Read the model definition and answer for the solid it produces. Units are mm, in the model's axes. Coordinates: 2 decimals unless noted, no trailing zeros.
Q1. Section A-A (x = 202) is taken. Count the separate pieces of the cut face and the enclosed holes in it, then the cut area to 3 significant figures.
Q2. Straight lines are drawn through the part: line 1 (Z direction, x = 544, y = 18); line 2 (Z direction, x = 88.5, y = -17); line 3 (Z direction, x = 320, y = 0). For each, find the intervals that lie inside material, in ascending order.
Q3. Flat-ended cylindrical pins translate along their axes: P1, Ø1, axis at x = 490.5, z = -3.5, coming from the +Y side; P2, Ø1.2, axis at x = 401.5, z = 1, coming from the +Y side. Find the tip coordinate at first contact, or state that the pin passes through.
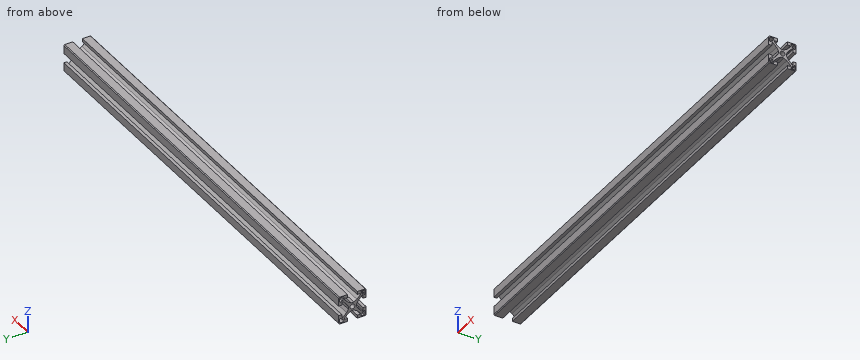
Autodesk Inventor part; units mm, degrees
ref_plane "CS_ANBAU_HINTEN_LINKS_XY" through (670, 0, 20) normal (1, 0, 0) x (0, 0, -1)
ref_plane "CS_ANBAU_HINTEN_LINKS_YZ" through (670, 0, 20) normal (0, 0, -1) x (0, 1, 0)
ref_plane "CS_ANBAU_HINTEN_LINKS_ZX" through (670, 0, 20) normal (0, 1, 0) x (1, 0, 0)
sketch "Skizze_1" plane through (0, 0, 0) normal (1, 0, 0) x (0, 1, 0)
  line L0 (18.75, 20) -> (7, 20)
  line L1 (7, 20) -> (7, 15.5)
  line L2 (7, 15.5) -> (11.7, 15.5)
  line L3 (11.7, 15.5) -> (11.7, 13.82)
  line L4 (11.7, 13.82) -> (6.4481, 8.5681)
  line L5 (6.4481, 8.5681) -> (2, 6)
  line L6 (2, 6) -> (-2, 6)
  line L7 (-2, 6) -> (-6.4481, 8.5681)
  line L8 (-6.4481, 8.5681) -> (-11.7, 13.82)
  line L9 (-11.7, 13.82) -> (-11.7, 15.5)
  line L10 (-11.7, 15.5) -> (-7, 15.5)
  line L11 (-7, 15.5) -> (-7, 20)
  line L12 (-7, 20) -> (-18.75, 20)
  line L13 (-18.75, 20) -> (-20, 18.75)
  line L14 (-20, 18.75) -> (-20, 7)
  line L15 (-20, 7) -> (-15.5, 7)
  line L16 (-15.5, 7) -> (-15.5, 11.7)
  line L17 (-15.5, 11.7) -> (-13.82, 11.7)
  line L18 (-13.82, 11.7) -> (-8.5681, 6.4481)
  line L19 (-8.5681, 6.4481) -> (-6, 2)
  line L20 (-6, 2) -> (-6, -2)
  line L21 (-6, -2) -> (-8.5681, -6.4481)
  line L22 (-8.5681, -6.4481) -> (-13.82, -11.7)
  line L23 (-13.82, -11.7) -> (-15.5, -11.7)
  line L24 (-15.5, -11.7) -> (-15.5, -7)
  line L25 (-15.5, -7) -> (-20, -7)
  line L26 (-20, -7) -> (-20, -18.75)
  line L27 (-20, -18.75) -> (-18.75, -20)
  line L28 (-18.75, -20) -> (-7, -20)
  line L29 (-7, -20) -> (-7, -15.5)
  line L30 (-7, -15.5) -> (-11.7, -15.5)
  line L31 (-11.7, -15.5) -> (-11.7, -13.82)
  line L32 (-11.7, -13.82) -> (-6.4481, -8.5681)
  line L33 (-6.4481, -8.5681) -> (-2, -6)
  line L34 (-2, -6) -> (2, -6)
  line L35 (2, -6) -> (6.4481, -8.5681)
  line L36 (6.4481, -8.5681) -> (11.7, -13.82)
  line L37 (11.7, -13.82) -> (11.7, -15.5)
  line L38 (11.7, -15.5) -> (7, -15.5)
  line L39 (7, -15.5) -> (7, -20)
  line L40 (7, -20) -> (18.75, -20)
  line L41 (18.75, -20) -> (20, -18.75)
  line L42 (20, -18.75) -> (20, -7)
  line L43 (20, -7) -> (15.5, -7)
  line L44 (15.5, -7) -> (15.5, -11.7)
  line L45 (15.5, -11.7) -> (13.82, -11.7)
  line L46 (13.82, -11.7) -> (8.5681, -6.4481)
  line L47 (8.5681, -6.4481) -> (6, -2)
  line L48 (6, -2) -> (6, 2)
  line L49 (6, 2) -> (8.5681, 6.4481)
  line L50 (8.5681, 6.4481) -> (13.82, 11.7)
  line L51 (13.82, 11.7) -> (15.5, 11.7)
  line L52 (15.5, 11.7) -> (15.5, 7)
  line L53 (15.5, 7) -> (20, 7)
  line L54 (20, 7) -> (20, 18.75)
  line L55 (20, 18.75) -> (18.75, 20)
  line L56 (17.75, -12.1) -> (17.1, -12.1)
  line L57 (17.1, -12.1) -> (15.45, -13.75)
  line L58 (15.45, -13.75) -> (14.5, -13.75)
  arc A0 (14.5, -13.75) -> (13.75, -14.5) centre (14.5, -14.5) ccw
  line L59 (13.75, -14.5) -> (13.75, -15.45)
  line L60 (13.75, -15.45) -> (12.1, -17.1)
  line L61 (12.1, -17.1) -> (12.1, -17.75)
  arc A1 (12.1, -17.75) -> (12.85, -18.5) centre (12.85, -17.75) ccw
  line L62 (12.85, -18.5) -> (17.5, -18.5)
  arc A2 (17.5, -18.5) -> (18.5, -17.5) centre (17.5, -17.5) ccw
  line L63 (18.5, -17.5) -> (18.5, -12.85)
  arc A3 (18.5, -12.85) -> (17.75, -12.1) centre (17.75, -12.85) ccw
  line L64 (-17.1, -12.1) -> (-17.75, -12.1)
  arc A4 (-17.75, -12.1) -> (-18.5, -12.85) centre (-17.75, -12.85) ccw
  line L65 (-18.5, -12.85) -> (-18.5, -17.5)
  arc A5 (-18.5, -17.5) -> (-17.5, -18.5) centre (-17.5, -17.5) ccw
  line L66 (-17.5, -18.5) -> (-12.85, -18.5)
  arc A6 (-12.85, -18.5) -> (-12.1, -17.75) centre (-12.85, -17.75) ccw
  line L67 (-12.1, -17.75) -> (-12.1, -17.1)
  line L68 (-12.1, -17.1) -> (-13.75, -15.45)
  line L69 (-13.75, -15.45) -> (-13.75, -14.5)
  arc A7 (-13.75, -14.5) -> (-14.5, -13.75) centre (-14.5, -14.5) ccw
  line L70 (-14.5, -13.75) -> (-15.45, -13.75)
  line L71 (-15.45, -13.75) -> (-17.1, -12.1)
  circle A8 centre (0, 0) radius 3.5
  arc A9 (-17.5, 18.5) -> (-18.5, 17.5) centre (-17.5, 17.5) ccw
  line L72 (-18.5, 17.5) -> (-18.5, 12.85)
  arc A10 (-18.5, 12.85) -> (-17.75, 12.1) centre (-17.75, 12.85) ccw
  line L73 (-17.75, 12.1) -> (-17.1, 12.1)
  line L74 (-17.1, 12.1) -> (-15.45, 13.75)
  line L75 (-15.45, 13.75) -> (-14.5, 13.75)
  arc A11 (-14.5, 13.75) -> (-13.75, 14.5) centre (-14.5, 14.5) ccw
  line L76 (-13.75, 14.5) -> (-13.75, 15.45)
  line L77 (-13.75, 15.45) -> (-12.1, 17.1)
  line L78 (-12.1, 17.1) -> (-12.1, 17.75)
  arc A12 (-12.1, 17.75) -> (-12.85, 18.5) centre (-12.85, 17.75) ccw
  line L79 (-12.85, 18.5) -> (-17.5, 18.5)
  line L80 (17.5, 18.5) -> (12.85, 18.5)
  arc A13 (12.85, 18.5) -> (12.1, 17.75) centre (12.85, 17.75) ccw
  line L81 (12.1, 17.75) -> (12.1, 17.1)
  line L82 (12.1, 17.1) -> (13.75, 15.45)
  line L83 (13.75, 15.45) -> (13.75, 14.5)
  arc A14 (13.75, 14.5) -> (14.5, 13.75) centre (14.5, 14.5) ccw
  line L84 (14.5, 13.75) -> (15.45, 13.75)
  line L85 (15.45, 13.75) -> (17.1, 12.1)
  line L86 (17.1, 12.1) -> (17.75, 12.1)
  arc A15 (17.75, 12.1) -> (18.5, 12.85) centre (17.75, 12.85) ccw
  line L87 (18.5, 12.85) -> (18.5, 17.5)
  arc A16 (18.5, 17.5) -> (17.5, 18.5) centre (17.5, 17.5) ccw
extrude "Extrusion1" add sketch "Skizze_1" along normal blind 670
ref_plane "CS_ANBAU_HINTEN_LINKS_XY" through (670, 0, 20) normal (1, 0, 0) x (0, 0, -1)
ref_plane "CS_ANBAU_HINTEN_LINKS_YZ" through (670, 0, 20) normal (0, 0, -1) x (0, 1, 0)
ref_plane "CS_ANBAU_HINTEN_LINKS_ZX" through (670, 0, 20) normal (0, 1, 0) x (1, 0, 0)
ref_plane "CS_ANBAU_HINTEN_OBEN_XY" through (670, 20, 0) normal (1, 0, 0) x (0, 0, -1)
ref_plane "CS_ANBAU_HINTEN_OBEN_YZ" through (670, 20, 0) normal (0, 0, -1) x (0, 1, 0)
ref_plane "CS_ANBAU_HINTEN_OBEN_ZX" through (670, 20, 0) normal (0, 1, 0) x (1, 0, 0)
ref_plane "CS_ANBAU_HINTEN_RECHTS_XY" through (670, 0, -20) normal (1, 0, 0) x (0, 0, -1)
ref_plane "CS_ANBAU_HINTEN_RECHTS_YZ" through (670, 0, -20) normal (0, 0, -1) x (0, 1, 0)
ref_plane "CS_ANBAU_HINTEN_RECHTS_ZX" through (670, 0, -20) normal (0, 1, 0) x (1, 0, 0)
ref_plane "CS_ANBAU_HINTEN_UNTEN_XY" through (670, -20, 0) normal (1, 0, 0) x (0, 0, -1)
ref_plane "CS_ANBAU_HINTEN_UNTEN_YZ" through (670, -20, 0) normal (0, 0, -1) x (0, 1, 0)
ref_plane "CS_ANBAU_HINTEN_UNTEN_ZX" through (670, -20, 0) normal (0, 1, 0) x (1, 0, 0)
ref_plane "CS_ANBAU_QUER_XY" through (0, 0, 20) normal (0, 0, 1) x (1, 0, 0)
ref_plane "CS_ANBAU_QUER_YZ" through (0, 0, 20) normal (1, 0, 0) x (0, 1, 0)
ref_plane "CS_ANBAU_QUER_ZX" through (0, 0, 20) normal (0, 1, 0) x (0, 0, 1)
ref_plane "CS_ANBAU_QUER_1_XY" through (670, 0, 20) normal (0, 0, 1) x (1, 0, 0)
ref_plane "CS_ANBAU_QUER_1_YZ" through (670, 0, 20) normal (1, 0, 0) x (0, 1, 0)
ref_plane "CS_ANBAU_QUER_1_ZX" through (670, 0, 20) normal (0, 1, 0) x (0, 0, 1)
ref_plane "CS_ANBAU_VORNE_LINKS_XY" through (0, 0, 20) normal (-1, 0, 0) x (0, 0, -1)
ref_plane "CS_ANBAU_VORNE_LINKS_YZ" through (0, 0, 20) normal (0, 0, -1) x (0, -1, 0)
ref_plane "CS_ANBAU_VORNE_LINKS_ZX" through (0, 0, 20) normal (0, -1, 0) x (-1, 0, 0)
ref_plane "CS_ANBAU_VORNE_OBEN_XY" through (0, 20, 0) normal (-1, 0, 0) x (0, 0, -1)
ref_plane "CS_ANBAU_VORNE_OBEN_YZ" through (0, 20, 0) normal (0, 0, -1) x (0, -1, 0)
ref_plane "CS_ANBAU_VORNE_OBEN_ZX" through (0, 20, 0) normal (0, -1, 0) x (-1, 0, 0)
ref_plane "CS_ANBAU_VORNE_RECHTS_XY" through (0, 0, -20) normal (-1, 0, 0) x (0, 0, -1)
ref_plane "CS_ANBAU_VORNE_RECHTS_YZ" through (0, 0, -20) normal (0, 0, -1) x (0, -1, 0)
ref_plane "CS_ANBAU_VORNE_RECHTS_ZX" through (0, 0, -20) normal (0, -1, 0) x (-1, 0, 0)
ref_plane "CS_ANBAU_VORNE_UNTEN_XY" through (0, -20, 0) normal (-1, 0, 0) x (0, 0, -1)
ref_plane "CS_ANBAU_VORNE_UNTEN_YZ" through (0, -20, 0) normal (0, 0, -1) x (0, -1, 0)
ref_plane "CS_ANBAU_VORNE_UNTEN_ZX" through (0, -20, 0) normal (0, -1, 0) x (-1, 0, 0)
ref_plane "p1_XY" through (0, 20, 0) normal (0, 0, 1) x (1, 0, 0)
ref_plane "p1_YZ" through (0, 20, 0) normal (1, 0, 0) x (0, 1, 0)
ref_plane "p1_ZX" through (0, 20, 0) normal (0, 1, 0) x (0, 0, 1)
ref_plane "p2_XY" through (670, 20, 0) normal (0, 0, 1) x (1, 0, 0)
ref_plane "p2_YZ" through (670, 20, 0) normal (1, 0, 0) x (0, 1, 0)
ref_plane "p2_ZX" through (670, 20, 0) normal (0, 1, 0) x (0, 0, 1)
ref_plane "p3_XY" through (670, -20, 18.75) normal (1, 0, 0) x (0, 0, -1)
ref_plane "p3_YZ" through (670, -20, 18.75) normal (0, 0, -1) x (0, 1, 0)
ref_plane "p3_ZX" through (670, -20, 18.75) normal (0, 1, 0) x (1, 0, 0)
ref_plane "p4_XY" through (670, 20, 18.75) normal (1, 0, 0) x (0, 0, -1)
ref_plane "p4_YZ" through (670, 20, 18.75) normal (0, 0, -1) x (0, 1, 0)
ref_plane "p4_ZX" through (670, 20, 18.75) normal (0, 1, 0) x (1, 0, 0)
ref_plane "p5_XY" through (670, 20, -21.25) normal (1, 0, 0) x (0, 0, -1)
ref_plane "p5_YZ" through (670, 20, -21.25) normal (0, 0, -1) x (0, 1, 0)
ref_plane "p5_ZX" through (670, 20, -21.25) normal (0, 1, 0) x (1, 0, 0)
ref_plane "pm1_XY" through (0, 0, 0) normal (1, 0, 0) x (0, 0, -1)
ref_plane "pm1_YZ" through (0, 0, 0) normal (0, 0, -1) x (0, 1, 0)
ref_plane "pm1_ZX" through (0, 0, 0) normal (0, 1, 0) x (1, 0, 0)
ref_plane "pm2_XY" through (670, 0, -1.25) normal (1, 0, 0) x (0, 0, -1)
ref_plane "pm2_YZ" through (670, 0, -1.25) normal (0, 0, -1) x (0, 1, 0)
ref_plane "pm2_ZX" through (670, 0, -1.25) normal (0, 1, 0) x (1, 0, 0)
properties part number "Robotunits Profil 40 x 40 - PIL 4040 SNN 0670"
Numbers:
1. separate pieces: 1
1. enclosed holes: 5
1. area: 564 mm2
2. line 1: z = -20 to -18.37, -12.14 to -7, 7 to 12.14, 18.37 to 20
2. line 2: z = -20 to -18.5, -12.2 to -7, 7 to 12.2, 18.5 to 20
2. line 3: z = -6 to -3.5, 3.5 to 6
3. P1: stops at y = 7.15
3. P2: stops at y = 6
